Source: CAD feature listing. Evaluate the final solid. Frame: model axes, mm. A direction names the side the tool comes from. Coordinates: 2 decimals unless noted, no trailing zeros. Loops run counter-clockwise (first coordinate to the right, second up) from the corner with the lowest first, then second, coordinate; pieces in that order, holes last.
from build123d import *

# Parameters (mm, degrees)
F0_W          = 42
F0_H          = 16
F1_DEPTH      = 133
F2_W          = 21
F2_H          = 52.7929635726
F3_DEPTH      = 20.1831926579
F4_W          = 21
F4_H          = 40.5876869309
F5_DEPTH      = 25
F6_W          = 90
F6_H          = 45.8940723884
F7_DEPTH      = 20.1831926579
F7_DEPTH_BACK = 25
F11_DEPTH     = 22
F13_DEPTH     = 25
F12_R         = 9.5
F14_DEPTH     = 25


with BuildPart() as f1:
    # F0 (on Front) → F1 (new body)
    with BuildSketch(Plane.XZ):
        with Locations((-0.8178073421, 8)):
            Rectangle(F0_W, F0_H)
        with BuildLine():
            Line((-21.8178073421, 27.5982314394), (-21.8178073421, 16))
            Line((-21.8178073421, 16), (20.1821926579, 16))
            Line((20.1821926579, 16), (20.1821926579, 27.5982314394))
            ThreePointArc((20.1821926579, 27.5982314394), (-0.8178073421, 48.5982314394), (-21.8178073421, 27.5982314394))
        make_face()
    extrude(amount=F1_DEPTH)

    # F2 (on Right) → F3 (cut, through all)
    with BuildSketch(Plane.YZ):
        with Locations((-122.5, 37.0988822573)):
            Rectangle(F2_W, F2_H)
    extrude(amount=F3_DEPTH, mode=Mode.SUBTRACT)

    # F4 (on face) → F5 (cut)
    with BuildSketch(Plane.YZ):
        with Locations((-122.5, 30.9962439364)):
            Rectangle(F4_W, F4_H)
    extrude(amount=-F5_DEPTH, mode=Mode.SUBTRACT)

    # F6 (on Right) → F7 (cut, two sides)
    with BuildSketch(Plane.YZ) as f7_sk:
        with Locations((-45, 33.6494366652)):
            Rectangle(F6_W, F6_H)
    extrude(amount=F7_DEPTH, mode=Mode.SUBTRACT)
    extrude(f7_sk.sketch, amount=-F7_DEPTH_BACK, mode=Mode.SUBTRACT)

    # F10 (on face) → F11 (join)
    with BuildSketch(Plane(origin=(-21.8178073421, 0, 0), x_dir=(0, -1, 0), z_dir=(-1, 0, 0))):
        with BuildLine():
            ThreePointArc((123.5257591727, 10.702400471), (118.6419482908, 35.6081422643), (108.6703372937, 58.9472630089))
            Line((108.6703372937, 58.9472630089), (22.1853906338, 10.702400471))
            Line((22.1853906338, 10.702400471), (90, 10.702400471))
            Line((90, 10.702400471), (90, 27.5982314394))
            Line((90, 27.5982314394), (112, 27.5982314394))
            Line((112, 27.5982314394), (112, 10.702400471))
            Line((112, 10.702400471), (123.5257591727, 10.702400471))
        make_face()
        with BuildLine():
            ThreePointArc((124, 0), (123.8813816514, 5.3564512553), (123.5257591727, 10.702400471))
            Line((123.5257591727, 10.702400471), (112, 10.702400471))
            Line((112, 10.702400471), (112, 27.5982314394))
            Line((112, 27.5982314394), (90, 27.5982314394))
            Line((90, 27.5982314394), (90, 10.702400471))
            Line((90, 10.702400471), (22.1853906338, 10.702400471))
            Line((22.1853906338, 10.702400471), (3, 0))
            Line((3, 0), (124, 0))
        make_face()
    extrude(amount=F11_DEPTH)

    # F8 (on face) → F13 (cut)
    with BuildSketch(Plane.XY.offset(10.702400471)):
        with BuildLine():
            ThreePointArc((6.5, -22.0442066215), (0, -15.5442066215), (-6.5, -22.0442066215))
            Line((-6.5, -22.0442066215), (-6.5, -66.0442066215))
            ThreePointArc((-6.5, -66.0442066215), (0, -72.5442066215), (6.5, -66.0442066215))
            Line((6.5, -66.0442066215), (6.5, -22.0442066215))
        make_face()
    extrude(amount=-F13_DEPTH, mode=Mode.SUBTRACT)

    # F12 (on face) → F14 (cut)
    with BuildSketch(Plane(origin=(0, -90, 0), x_dir=(-1, 0, 0), z_dir=(0, 1, 0))):
        with Locations((0, 32.2404283148)):
            Circle(F12_R)
    extrude(amount=-F14_DEPTH, mode=Mode.SUBTRACT)


solid = f1.part
Q1. Contact query for flat-ended pins moving along their axis: pin 1 Ø10 at (x, z) = (-34, 51) entering from -Y; pin 2 Ø6 at (x, z) = (-12.5, 27) entering from -Y; pin 3 Ø3 at (x, z) = (-16.5, 21) entering from +Y; pin 4 Ø1 at (x, y) = (8, -34.5) entering from -Z. Output: stop coordinate, or through.
Q2. Section D-D, the plane y = -106.5. Return the cut outline in (x, z), plus the area to 3 significant figures.
Q3. Draft query along Z for faces 1 (the cylindrical face through (2.059, -100.846, 22.966)), 2 (the flat face through (-11, -66, 0)), 3 (the cylindrical face through (-0.143, -72.543, 5.426)). Return one class per face: +Z half, -Z half, draft (parallel to the pull), parting line (faces both ways), or undercut.
Q4. Access query for faces 4 (the cylindrical face through (0.143, -15.546, 5.426)), 5 (the flat face through (9, -46, 10.702)), 6 (the flat face through (-21.818, -8, 7)), 7 (the flat face through (-1, -123, 10.702)). Directions: +Z, -Z, +X, -X, +Y, -Y. A direction counts if a zero-diameter tool reaches every point of the face in a straight line with its end or side. Return the directions, or none.
Q5. Section C-C, the plane z = 18. Return the cut outline in (x, y).
Q6. Line query: line 1 along Z through (x, y) = (0, -106.5); line 2 along Y through (x, z) = (-0.5, 9.5); line 3 along X through (y, z) = (-78, 12.5). Output: solid intervals per line, ascending.
Q7. Section B-B, the plane x = 0. Return the cut outline in (y, z).
Q8. Section A-A, the plane y = -20. Return the cut outline in (x, z), plus the area to 3 significant figures.
Derived:
1. pin 1: stops at y = -114.92
1. pin 2: stops at y = -112
1. pin 3: stops at y = -90
1. pin 4: stops at z = 0
2. outline: (-43.82, 0) - (20.18, 0) - (20.18, 27.6) arc R21 ccw to (-21.82, 27.6) - (-21.82, 57.74) - (-43.82, 57.74) - close; hole circle Ø19 at (0, 32.24)
2. area: 2,840 mm2
3. face 1: undercut
3. face 2: -Z half
3. face 3: draft
4. face 4: +Z, -Z
4. face 5: +Z, +X, +Y
4. face 6: +Z, -X, +Y
4. face 7: +Z, +X, -Y
5. outline: (-43.82, -122.65) - (-21.82, -122.65) - (-21.82, -112) - (20.18, -112) - (20.18, -90) - (-21.82, -90) - (-21.82, -35.27) - (-43.82, -35.27) - close
6. line 1: z = 0 to 22.74, 41.74 to 48.58
6. line 2: y = -133 to -72.52, -15.56 to 0
6. line 3: x = -43.82 to -21.82
7. outline: (-133, 0) - (-72.54, 0) - (-72.54, 10.7) - (-90, 10.7) - (-90, 22.74) - (-112, 22.74) - (-112, 10.7) - (-133, 10.7) - close; (-112, 41.74) - (-90, 41.74) - (-90, 48.58) - (-112, 48.58) - close; (-15.54, 0) - (0, 0) - (0, 10.7) - (-15.54, 10.7) - close
8. outline: (-43.82, 0) - (-6.17, 0) - (-6.17, 10.7) - (-21.82, 10.7) - (-21.82, 9.48) - (-43.82, 9.48) - close; (6.17, 0) - (20.18, 0) - (20.18, 10.7) - (6.17, 10.7) - close
8. area: 526 mm2
